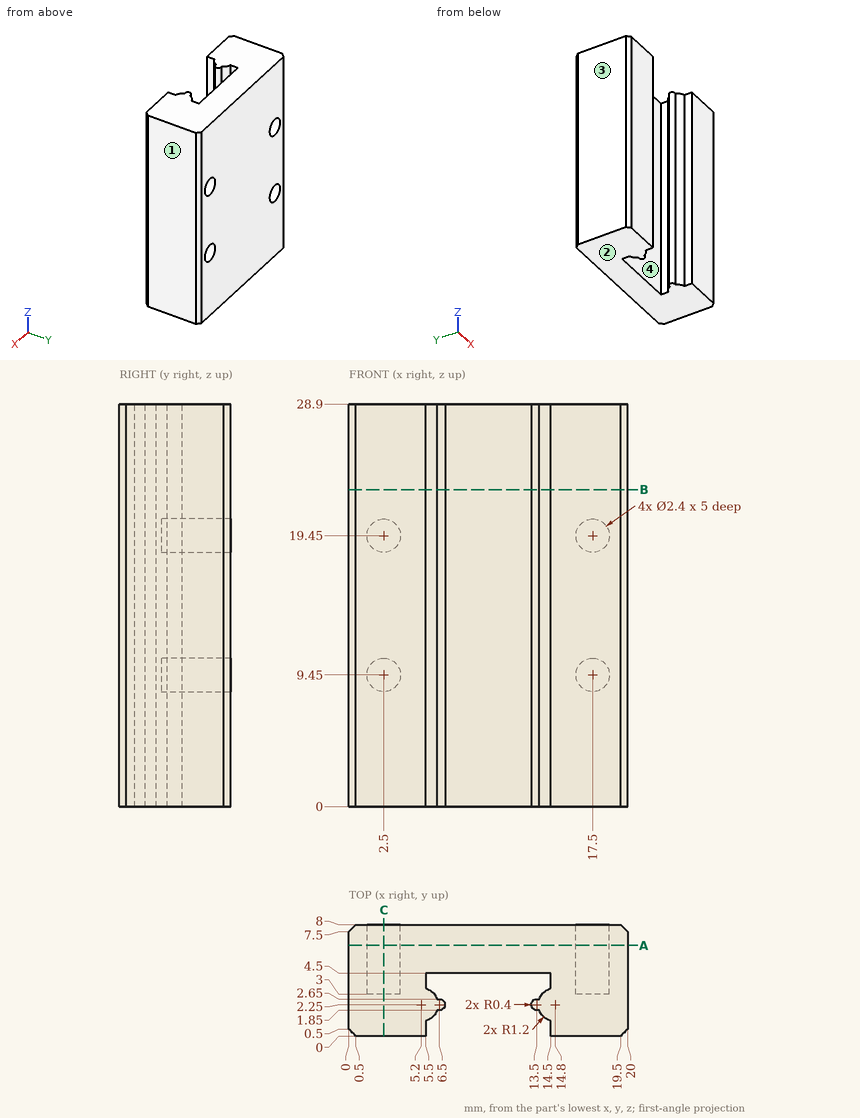
The drawing under review shows one solid part. Ordinate dimensions are in mm from its lowest x, y, z. Round coordinates to 2 decimals unless told otherwise and drop trailing zeros. Write each loop counter-clockwise with the first axis right and the second up, starting at its lowest first coordinate (ties: lowest second). Pieces come first, ordered by that corner, then holes. Notation, with made-up numbers: (50.5, 71.25) - (106.5, 71.25) arc R20 ccw to (106.5, 100.25) - close; hole circle Ø6 at (58, -14.75). An arc over 180 degrees is marked (long way). Put each result on its own line as item: value.
Q1. We need section B-B (z = 22.75). Give the boundary of the cut face in (x, y).
Solved:
outline: (0, 0.5) - (0.5, 0) - (5.5, 0) - (5.5, 1.09) arc R1.2 ccw to (6.33, 1.85) - (6.5, 1.85) arc R0.4 ccw to (6.5, 2.65) - (6.33, 2.65) arc R1.2 ccw to (5.5, 3.41) - (5.5, 4.5) - (14.5, 4.5) - (14.5, 3.41) arc R1.2 ccw to (13.67, 2.65) - (13.5, 2.65) arc R0.4 ccw to (13.5, 1.85) - (13.67, 1.85) arc R1.2 ccw to (14.5, 1.09) - (14.5, 0) - (19.5, 0) - (20, 0.5) - (20, 7.5) - (19.5, 8) - (0.5, 8) - (0, 7.5) - close
Q2. Mouldability with a two-part tool opening along X and no side actions: class the marked faces 1, 2, 3 and 4 as released by +X, released by -X, zero draft, split by the parting line, or undercut.
Solved:
face 1: released by +X
face 2: zero draft
face 3: released by -X
face 4: undercut
Q3. Wall thickness on probe 1 along X at (y, z) = (4.9, 9.45); probe 2 along X at (y, z) = (4, 27); probe 3 along Y at (x, z) = (9.25, 19.25): over which ranges is each line inside the solid? List them lowest first.
Solved:
probe 1: x = 0 to 1.3, 3.7 to 16.3, 18.7 to 20
probe 2: x = 0 to 5.5, 14.5 to 20
probe 3: y = 4.5 to 8
Q4. We need section A-A (y = 6.5). Give the boundary of the cut face in (x, z), and give its area (3 significant figures).
Solved:
outline: (0, 0) - (20, 0) - (20, 28.9) - (0, 28.9) - close; hole circle Ø2.4 at (2.5, 9.45); hole circle Ø2.4 at (2.5, 19.45); hole circle Ø2.4 at (17.5, 9.45); hole circle Ø2.4 at (17.5, 19.45)
area: 560 mm2
Q5. Insertion check: pin 1 Ø2.5 at (x, z) = (11.5, 18) entering from -Y; pin 2 Ø2.5 at (x, z) = (18, 20) entering from +Y; pin 3 Ø1.4 at (x, z) = (2.5, 9.45) entering from +Y. Each pin has a flat end and moves straight along its axis. Give the tip position at first contact, or say it passes through.
Solved:
pin 1: stops at y = 4.5
pin 2: stops at y = 8
pin 3: stops at y = 3
Q6. We need section C-C (x = 2.5). Give the boundary of the cut face in (y, z).
Solved:
outline: (0, 0) - (8, 0) - (8, 8.25) - (3, 8.25) - (3, 10.65) - (8, 10.65) - (8, 18.25) - (3, 18.25) - (3, 20.65) - (8, 20.65) - (8, 28.9) - (0, 28.9) - close
